from build123d import *

# Parameters (mm, degrees)
SKETCH1_W           = 60
SKETCH1_H           = 50
BASE_FLANGE1_DEPTH  = 5
SKETCH6_R           = 5
CUT_EXTRUDE1_DEPTH  = 66.192024052
EDGE_FLANGE1_DEPTH  = 50
HOLE1_START         = 5
HOLE1_OUTLINE_R     = 2.5
HOLE1_DEPTH         = 5
LPATTERN1_COUNT     = 2
LPATTERN1_PITCH     = 15
LPATTERN1_COL_COUNT = 2
LPATTERN1_COL_PITCH = 15


# Read off the part's stored shape, not the designer's step: Hole1
# Sheet-metal steps are written as plain solids
with BuildPart() as part:
    # Sketch1 → Base-Flange1 (new body)
    with BuildSketch(Plane.XY):
        with Locations((-30, 0)):
            Rectangle(SKETCH1_W, SKETCH1_H)
    extrude(amount=-BASE_FLANGE1_DEPTH)

    # Sketch6 → Cut-Extrude1 (cut, through all)
    with BuildSketch(Plane.XY):
        with Locations((-45, 0)):
            Circle(SKETCH6_R)
        with Locations((-15, 0)):
            Circle(SKETCH6_R)
    extrude(amount=-CUT_EXTRUDE1_DEPTH, mode=Mode.SUBTRACT)

    # Edge-Flange1 section (across the edge) → Edge-Flange1 (add)
    with BuildSketch(Plane(origin=(5, -25, 0), x_dir=(-1, 0, 0), z_dir=(0, 1, 0))):
        with BuildLine():
            Line((-5, 5), (-5, 25))
            Line((-5, 25), (0, 25))
            Line((0, 25), (0, 5))
            ThreePointArc((0, 5), (1.464466094, 1.464466094), (5, 0))
            Line((5, 0), (5, -5))
            ThreePointArc((5, -5), (-2.071067812, -2.071067812), (-5, 5))
        make_face()
    extrude(amount=EDGE_FLANGE1_DEPTH)

    # Hole1 outline → Hole1 (cut)
    with BuildSketch(Plane.YZ.offset(HOLE1_START)):
        with Locations((0, 10)):
            Circle(HOLE1_OUTLINE_R)
    hole1 = extrude(amount=HOLE1_DEPTH, mode=Mode.SUBTRACT)

    # LPattern1: Hole1 ×2
    with Locations(*[(0, i * LPATTERN1_PITCH, 0) for i in range(1, LPATTERN1_COUNT)]):
        add(hole1, mode=Mode.SUBTRACT)

    # LPattern1 col: Hole1 ×2
    with Locations(*[(0, -i * LPATTERN1_COL_PITCH, 0) for i in range(1, LPATTERN1_COL_COUNT)]):
        add(hole1, mode=Mode.SUBTRACT)


solid = part.part
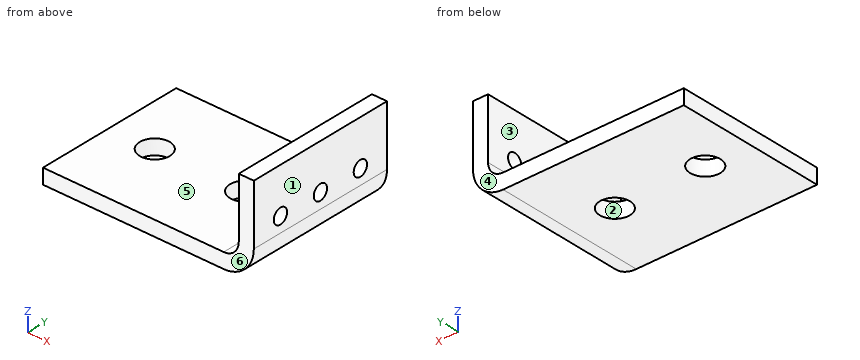
CAD build for the part. Positions are in the model's coordinates, mm. Face numbers are marked on the shaded views. A direction names the side the tool comes from. Coordinates: 2 decimals unless noted, no trailing zeros. Order: outer loops, then holes, each group sorted by start corner. A loop starts at its lowest first (then second) coordinate and runs counter-clockwise, first axis right, second up.
Item 1: 3-axis set-ups, long thin cutter, end or side, ignore diameter. For the marked faces 5 and 6: which of +Z, -Z, +X, -X, +Y, -Y reach the whole face in a straight line?
Check sheet entries:
face 5: +Z, -X, +Y, -Y
face 6: +Z, -Z, +X, -X, -Y
Item 2: Drill centre lines: L1, parallel to X at y = 8, z = 17.25; L2, parallel to Z at x = -11.5, y = 10; L3, parallel to Z at x = 6.3, y = 15. Where is each one in solid material? Low to high.
Check sheet entries:
L1: x = 5 to 10
L2: z = -5 to 0
L3: z = -2.77 to 7.5, 12.5 to 25
Item 3: Band-saw the part on A-A on x = -18. List the corners of the cut face in (y, z).
Check sheet entries:
outline: (-25, -5) - (-4, -5) - (-4, 0) - (-25, 0) - close; (4, -5) - (25, -5) - (25, 0) - (4, 0) - close
Item 4: Band-saw the part on D-D on y = 0. List the corners of the cut face in (x, z).
Check sheet entries:
outline: (-60, -5) - (-50, -5) - (-50, 0) - (-60, 0) - close; (-40, -5) - (-20, -5) - (-20, 0) - (-40, 0) - close; (-10, -5) - (0, -5) arc R10 ccw to (10, 5) - (10, 7.5) - (5, 7.5) - (5, 5) arc R5 cw to (0, 0) - (-10, 0) - close; (5, 12.5) - (10, 12.5) - (10, 25) - (5, 25) - close
Item 5: Band-saw the part on C-C on y = -15. List the corners of the cut face in (x, z).
Check sheet entries:
outline: (-60, -5) - (0, -5) arc R10 ccw to (10, 5) - (10, 7.5) - (5, 7.5) - (5, 5) arc R5 cw to (0, 0) - (-60, 0) - close; (5, 12.5) - (10, 12.5) - (10, 25) - (5, 25) - close
Item 6: Band-saw the part on B-B on z = 10. List the corners of the cut face in (x, y), plus the area to 3 significant figures.
Check sheet entries:
outline: (5, -25) - (10, -25) - (10, -17.5) - (5, -17.5) - close; (5, -12.5) - (10, -12.5) - (10, -2.5) - (5, -2.5) - close; (5, 2.5) - (10, 2.5) - (10, 12.5) - (5, 12.5) - close; (5, 17.5) - (10, 17.5) - (10, 25) - (5, 25) - close
area: 175 mm2
Item 7: Pin check, flat tip, straight feed: pin 1 Ø6 at (y, z) = (-15, 10) entering from -X. Stop position of the tip, or through.
Check sheet entries:
pin 1: stops at x = 5
Item 8: Two-plate mould, pull along X, no slides. Class the marked faces 1, 2, 3 and 4: +X half, -X half, draft (parallel to the pull), parting line (faces both ways), or undercut.
Check sheet entries:
face 1: +X half
face 2: undercut
face 3: -X half
face 4: draft
